Model file for the job. Use its own axes, mm. Face numbers are marked on the shaded views. A direction names the side the tool comes from. Give positions to 0.01 mm unless a question says otherwise; leave off trailing zeros. Loops run counter-clockwise (first coordinate to the right, second up) from the corner with the lowest first, then second, coordinate; pieces in that order, holes last. Notation, with made-up numbers: (-2, 47.25) - (21, 47.25) arc R8 ccw to (21, 59.25) - close; hole circle Ø1 at (6.5, 38). An arc over 180 degrees is marked (long way). Use a Markdown table: item, result.
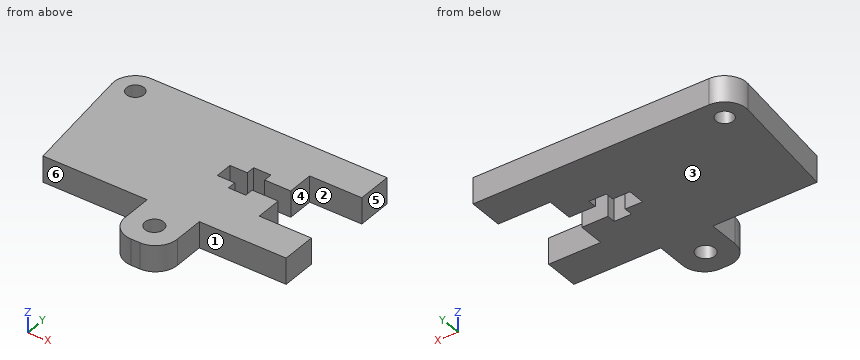
from build123d import *

# Parameters (mm, degrees)
F0_R     = 2.734931
F0_R_2   = 2.544482
F1_DEPTH = 7.62


with BuildPart() as f1:
    # F0 (on Top) → F1 (new body)
    with BuildSketch(Plane.XY):
        with BuildLine():
            Line((15.24, 42.192222), (-53.766833, 42.192222))
            ThreePointArc((-53.766833, 42.192222), (-58.527289, 40.044669), (-60.067797, 35.054602))
            Line((-60.067797, 35.054602), (-55.88, 1.552223))
            Line((-55.88, 1.552223), (-25.4, 1.552223))
            Line((-25.4, 1.552223), (-25.4, -7.337777))
            ThreePointArc((-25.4, -7.337777), (-23.540128, -11.827905), (-19.05, -13.687777))
            Line((-19.05, -13.687777), (-16.51, -13.687777))
            ThreePointArc((-16.51, -13.687777), (-12.019872, -11.827905), (-10.16, -7.337777))
            Line((-10.16, -7.337777), (-10.16, 1.552223))
            Line((-10.16, 1.552223), (15.24, 1.552223))
            Line((15.24, 1.552223), (15.24, 11.712223))
            Line((15.24, 11.712223), (0, 11.712223))
            Line((0, 11.712223), (0, 19.332223))
            Line((0, 19.332223), (-7.62, 19.332223))
            Line((-7.62, 19.332223), (-7.62, 16.792223))
            Line((-7.62, 16.792223), (-12.7, 16.792223))
            Line((-12.7, 16.792223), (-12.7, 19.332223))
            Line((-12.7, 19.332223), (-17.78, 19.332223))
            Line((-17.78, 19.332223), (-17.78, 24.412223))
            Line((-17.78, 24.412223), (-12.7, 24.412223))
            Line((-12.7, 24.412223), (-12.7, 26.952223))
            Line((-12.7, 26.952223), (-7.62, 26.952223))
            Line((-7.62, 26.952223), (-7.62, 24.412223))
            Line((-7.62, 24.412223), (0, 24.412223))
            Line((0, 24.412223), (0, 32.032222))
            Line((0, 32.032222), (15.24, 32.032222))
            Line((15.24, 32.032222), (15.24, 42.192222))
        make_face()
        with Locations((-17.78, -6.067777)):
            Circle(F0_R, mode=Mode.SUBTRACT)
        with Locations((-53.766833, 35.842222)):
            Circle(F0_R_2, mode=Mode.SUBTRACT)
    extrude(amount=F1_DEPTH)


solid = f1.part
(1) 3-axis set-ups, long thin cutter, end or side, ignore diameter. For the marked faces 1, 2 and 3: which of +Z, -Z, +X, -X, +Y, -Y reach the whole face in a straight line?
Computed:
| item | result |
|---|---|
| face 1 | +Z, -Z, +X, -Y |
| face 2 | +Z, -Z, +X |
| face 3 | -Z, +X, -X, +Y, -Y |
(2) Slice it at A-A, the plane x = 1. Write the cut outline in (y, z), plus the area to 3 significant figures.
Computed:
| item | result |
|---|---|
| outline | (1.55, 0) - (11.71, 0) - (11.71, 7.62) - (1.55, 7.62) - close; (32.03, 0) - (42.19, 0) - (42.19, 7.62) - (32.03, 7.62) - close |
| area | 155 mm² |
(3) Slice it at C-C, the plane x = -46.5. Write the cut outline in (y, z), plus the area to 3 significant figures.
Computed:
| item | result |
|---|---|
| outline | (1.55, 0) - (42.19, 0) - (42.19, 7.62) - (1.55, 7.62) - close |
| area | 310 mm² |
(4) Pin check, flat tips, straight feed: P1, Ø2, axis at y = -4, z = 5.5, coming from the -X side; P2, Ø2.5, axis at x = -36.5, z = 2.5, coming from the -Y side; P3, Ø1.3, axis at y = 26.5, z = 5, coming from the -X side. Stop position of each tip, or through.
Computed:
| item | result |
|---|---|
| P1 | x = -25.4 |
| P2 | y = 1.55 |
| P3 | x = -59.08 |
(5) Mould opens along Y. For the marked faces 4, 5 and 6 say: pulls with the +Y half, pulls with the -Y half, needs draft (parallel to the pull), parting line crosses it, or undercut.
Computed:
| item | result |
|---|---|
| face 4 | undercut |
| face 5 | needs draft |
| face 6 | pulls with the -Y half |
(6) Slice it at D-D, the plane y = 7. Write the cut outline in (x, z), plus the area to 3 significant figures.
Computed:
| item | result |
|---|---|
| outline | (-56.56, 0) - (15.24, 0) - (15.24, 7.62) - (-56.56, 7.62) - close |
| area | 547 mm² |
(7) Slice it at B-B, the plane z = 6.75. Count the separate pieces of the cut face and the enclosed holes in it, plus the area to 3 significant figures.
Computed:
| item | result |
|---|---|
| separate pieces | 1 |
| enclosed holes | 2 |
| area | 2,730 mm² |
(8) Drill centre lines: probe 1 along Y at (x, z) = (2, 3); probe 2 along Y at (x, z) = (-3.5, 3.25); probe 3 along X at (y, z) = (-6, 3.5). Where is each one in solid material? Low to high. Write a range as [from, to].
Computed:
| item | result |
|---|---|
| probe 1 | [1.55, 11.71], [32.03, 42.19] |
| probe 2 | [1.55, 19.33], [24.41, 42.19] |
| probe 3 | [-25.4, -20.51], [-15.05, -10.16] |
